Input: part model. Units: mm. Frame: model coordinates. A direction names the side the tool comes from. Give positions to 0.01 mm unless a question says otherwise; leave off trailing zeros. Write each loop counter-clockwise with the first axis right and the second up, starting at its lowest first coordinate (ties: lowest second). Pieces come first, ordered by that corner, then holes.
```python
from build123d import *

# Parameters (mm, degrees)
SKETCH1_R                = 0.6
BOSS_EXTRUDE1_DEPTH      = 0.5
BOSS_EXTRUDE1_DEPTH_BACK = 0.5


with BuildPart() as part:
    # Sketch1 → Boss-Extrude1 (new body, two sides)
    with BuildSketch(Plane(origin=(0, 0, 0), x_dir=(0, 0, -1), z_dir=(1, 0, 0))) as boss_extrude1_sk:
        with BuildLine():
            Line((-1.575903864, -5.685642181), (-0.792131706, -4.328108982))
            ThreePointArc((-0.792131706, -4.328108982), (-1.835210176, -2.355544978), (-3.685531471, -3.602674702))
            ThreePointArc((-3.685531471, -3.602674702), (0, 4.4), (3.685531471, -3.602674702))
            ThreePointArc((3.685531471, -3.602674702), (1.835210176, -2.355544978), (0.792131706, -4.328108982))
            Line((0.792131706, -4.328108982), (1.575903864, -5.685642181))
            ThreePointArc((1.575903864, -5.685642181), (0, 5.9), (-1.575903864, -5.685642181))
        make_face()
        with Locations((2.2, -3.810511777)):
            Circle(SKETCH1_R, mode=Mode.SUBTRACT)
        with Locations((-2.2, -3.810511777)):
            Circle(SKETCH1_R, mode=Mode.SUBTRACT)
    extrude(amount=BOSS_EXTRUDE1_DEPTH)
    extrude(boss_extrude1_sk.sketch, amount=-BOSS_EXTRUDE1_DEPTH_BACK)


solid = part.part
```
Item 1: Mould query, pull axis Z, two halves, no side actions, for faces 1 (the cylindrical face through (0.007, 5.895, -0.237)), 2 (the flat face through (-0.5, -2.9, 1.3)), 3 (the cylindrical face through (-0.01, -4.34, -2.48)). Classes: +Z half, -Z half, draft (parallel to the pull), parting line (faces both ways), or undercut.
Item 2: Section C-C (x = -0.05). Return loops of the section in (y, z), and give its area (3 significant figures).
Item 3: Set-up query: faces 4 (the flat face through (0.01, -5, -1.18)), 5 (the flat face through (0.5, -2.9, 1.3)). Return all of +Z, -Z, +X, -X, +Y, -Y with unobstructed straight access to the full face (end or side cutting, diameter ignored); none if empty.
Item 4: Pin query (flat end, axial travel): pin 1 (1 mm diameter, centred on y = -3.81, z = -2.2, fed in from +X). Return the tip coordinate at first contact, or that it passes through.
Item 5: Section B-B (y = 0). Return loops of the section in (x, z), and give its area (3 significant figures).
Item 6: Section D-D (z = -2.25). Return loops of the section in (x, y).
Item 7: Section A-A (z = 4.5). Return loops of the section in (x, y), and give its area (3 significant figures).
Item 8: Ray query, line 1 (Z direction, x = -0.1, y = -4); line 2 (Y direction, x = -0.25, z = -2.2); line 3 (Z direction, x = -0.4, y = -3). Return the intervals inside material, ascending.
Solved:
1. face 1: parting line
1. face 2: draft
1. face 3: undercut
2. outline: (-5.69, -1.58) arc R5.9 ccw (long way) to (-5.69, 1.58) - (-4.33, 0.79) arc R1.5 ccw (long way) to (-3.6, 3.69) arc R4.85 cw (long way) to (-3.6, -3.69) arc R1.5 ccw (long way) to (-4.33, -0.79) - close; hole circle Ø1.2 at (-3.81, -2.2); hole circle Ø1.2 at (-3.81, 2.2)
2. area: 43.0 mm2
3. face 4: +X, -X, -Y
3. face 5: +Z, -Z, +X, +Y, -Y
4. pin 1: passes through
5. outline: (-0.5, -5.9) - (0.5, -5.9) - (0.5, -4.83) - (-0.5, -4.83) - close; (-0.5, 4.83) - (0.5, 4.83) - (0.5, 5.9) - (-0.5, 5.9) - close
5. area: 2.14 mm2
6. outline: (-0.5, -5.45) - (0.5, -5.45) - (0.5, -4.41) - (-0.5, -4.41) - close; (-0.5, -3.21) - (0.5, -3.21) - (0.5, -2.31) - (-0.5, -2.31) - close; (-0.5, 3.85) - (0.5, 3.85) - (0.5, 5.45) - (-0.5, 5.45) - close
7. outline: (-0.5, -3.82) - (0.5, -3.82) - (0.5, -2.26) - (-0.5, -2.26) - close; (-0.5, 1.36) - (0.5, 1.36) - (0.5, 3.82) - (-0.5, 3.82) - close
7. area: 4.01 mm2
8. line 1: z = -4.34 to -2.77, -1.63 to -0.71, 0.71 to 1.63, 2.77 to 4.34
8. line 2: y = -5.47 to -4.41, -3.21 to -2.31, 3.87 to 5.47
8. line 3: z = -5.08 to -4.13, -3.46 to -0.94, 0.94 to 3.46, 4.13 to 5.08
